```python
from build123d import *

# Parameters (mm, degrees)
SKETCH_W  = 97.5
SKETCH_H  = 50
SKETCH_R  = 1.4
PAD_DEPTH = 2
FILLET_R  = 1


with BuildPart() as part:
    # Sketch → Pad (new body)
    with BuildSketch(Plane.XY):
        Rectangle(SKETCH_W, SKETCH_H)
        with Locations((-45.75, 22)):
            Circle(SKETCH_R, mode=Mode.SUBTRACT)
        with Locations((45.75, 22)):
            Circle(SKETCH_R, mode=Mode.SUBTRACT)
        with Locations((45.75, -22)):
            Circle(SKETCH_R, mode=Mode.SUBTRACT)
        with Locations((-45.75, -22)):
            Circle(SKETCH_R, mode=Mode.SUBTRACT)
    extrude(amount=PAD_DEPTH)

    # Fillet
    fillet_edges = [part.edges().sort_by_distance(p)[0] for p in [
        (48.75, 0, 2),
        (48.75, 25, 1),
        (48.75, -25, 1),
        (0, -25, 2),
        (0, 25, 2),
        (-48.75, 0, 2),
        (-48.75, 25, 1),
        (-48.75, -25, 1),
    ]]
    fillet(fillet_edges, radius=FILLET_R)


solid = part.part
```
Geometry check sheet. Reference: the model listing, model coordinates, mm. Give positions to 0.01 mm unless a question says otherwise; leave off trailing zeros. Write each loop counter-clockwise with the first axis right and the second up, starting at its lowest first coordinate (ties: lowest second). Pieces come first, ordered by that corner, then holes. Notation, with made-up numbers: (-23.75, -11.5) - (10.25, -11.5) arc R15 ccw to (10.25, 4.5) - close; hole circle Ø3 at (6.5, 50.25). An arc over 180 degrees is marked (long way). Use a Markdown table: item, result.
Q1. Section check B-B, the plane x = 45.75. Enter the section's corners in (y, z), then the cut area to 3 significant figures.
Computed:
| item | result |
|---|---|
| outline | (-25, 0) - (-23.4, 0) - (-23.4, 2) - (-24, 2) arc R1 ccw to (-25, 1) - close; (-20.6, 0) - (20.6, 0) - (20.6, 2) - (-20.6, 2) - close; (23.4, 0) - (25, 0) - (25, 1) arc R1 ccw to (24, 2) - (23.4, 2) - close |
| area | 88.4 mm² |
Q2. Draft check along Y on faces 1 (the face through (-45.1, 20.76, 0.99)), 2 (the face through (-1, 0, 2)). Enter one of: pulls with the +Y half, pulls with the -Y half, needs draft (parallel to the pull), parting line crosses it, or undercut.
Computed:
| item | result |
|---|---|
| face 1 | undercut |
| face 2 | needs draft |
Q3. Thickness scan on L1, parallel to Y at x = -45.75, z = 0.95; L2, parallel to Y at x = 45.75, z = 1.5; L3, parallel to X at y = -18.5, z = 1.8. Record the ranges inside material, lowest first. Write a range as [from, to].
Computed:
| item | result |
|---|---|
| L1 | y = [-25, -23.4], [-20.6, 20.6], [23.4, 25] |
| L2 | y = [-24.87, -23.4], [-20.6, 20.6], [23.4, 24.87] |
| L3 | x = [-48.35, 48.35] |
Q4. Section check A-A, the plane y = -22. Enter the section's corners in (x, z).
Computed:
| item | result |
|---|---|
| outline | (-48.75, 0) - (-47.15, 0) - (-47.15, 2) - (-47.75, 2) arc R1 ccw to (-48.75, 1) - close; (-44.35, 0) - (44.35, 0) - (44.35, 2) - (-44.35, 2) - close; (47.15, 0) - (48.75, 0) - (48.75, 1) arc R1 ccw to (47.75, 2) - (47.15, 2) - close |
